Autodesk Inventor part; units mm, degrees
ref_plane "YZ Plane" through (0, 0, 0) normal (1, 0, 0) x (0, 1, 0)
ref_plane "XZ Plane" through (0, 0, 0) normal (0, 1, 0) x (-1, 0, 0)
ref_plane "XY Plane" through (0, 0, 0) normal (0, 0, 1) x (1, 0, 0)
sketch "Sketch1" plane through (0, 0, 0) normal (0, 1, 0) x (-1, 0, 0)
  circle A0 centre (0, 0) radius 12.7
  dimension "d0" = 25.4
extrude "Extrusion1" add sketch "Sketch1" along normal blind 3
sketch "Sketch2" plane through (0, 3, 0) normal (0, 1, 0) x (1, 0, 0)
  circle A0 centre (0, 0) radius 7.125
  dimension "d3" = 14.25
extrude "Extrusion2" add sketch "Sketch2" along normal blind 3
sketch "Sketch3" plane through (0, 6, 0) normal (0, 1, 0) x (1, 0, 0)
  circle A0 centre (0, 0) radius 2.54
  dimension "d6" = 5.08
extrude "Extrusion3" cut sketch "Sketch3" against normal up to next
properties part number "PhotonCerberCageInsert"
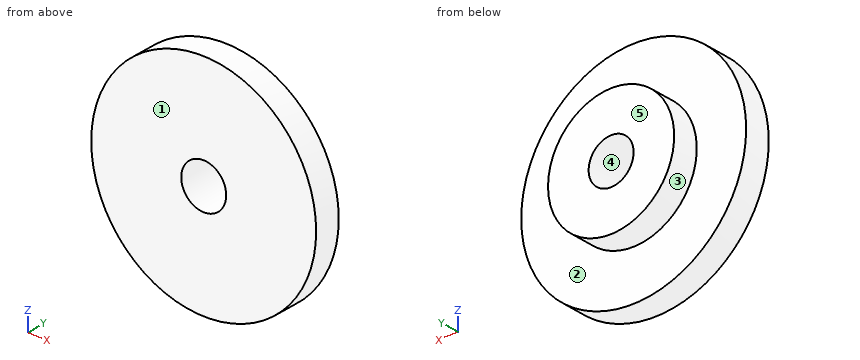
Geometry: final body of the model. Coordinates: model frame, mm. Face numbers are marked on the shaded views. A direction names the side the tool comes from. Give positions to 0.01 mm unless a question says otherwise; leave off trailing zeros. Write each loop counter-clockwise with the first axis right and the second up, starting at its lowest first coordinate (ties: lowest second). Pieces come first, ordered by that corner, then holes. Notation, with made-up numbers: (-22.75, -10.5) -> (21.25, -10.5) arc R6 cw to (21.25, -6.5) -> close; hole circle Ø6 at (-3, 14.25). An arc over 180 degrees is marked (long way). Answer as a JSON object with one key per item and string values.
1. Cut plane C-C on y = 2.5. Output: boundary loops of the cut face in (x, z).
Ans:
{"outline": "circle Ø25.4 at (0, 0); hole circle Ø5.08 at (0, 0)"}
2. Mould query, pull axis X, two halves, no side actions, for the marked faces 3, 4 and 5. Classes: pulls with the +X half, pulls with the -X half, needs draft (parallel to the pull), parting line crosses it, or undercut.
Ans:
{"face 3": "parting line crosses it", "face 4": "undercut", "face 5": "needs draft"}
3. Cut plane D-D on z = 5.5. Output: boundary loops of the cut face in (x, y), and give its area (3 significant figures).
Ans:
{"outline": "(-11.45, 0) -> (11.45, 0) -> (11.45, 3) -> (4.53, 3) -> (4.53, 6) -> (-4.53, 6) -> (-4.53, 3) -> (-11.45, 3) -> close", "area": "95.9 mm^2"}
4. Cut plane B-B on x = -1.5. Output: boundary loops of the cut face in (y, z).
Ans:
{"outline": "(0, -12.61) -> (3, -12.61) -> (3, -6.97) -> (6, -6.97) -> (6, -2.05) -> (0, -2.05) -> close; (0, 2.05) -> (6, 2.05) -> (6, 6.97) -> (3, 6.97) -> (3, 12.61) -> (0, 12.61) -> close"}
5. Contact query for a flat-ended pin moving along its axis: pin 1 (2 mm diameter, centred on x = -4, y = 2.5, fed in from +Z). Output: stop coordinate, or through.
Ans:
{"pin 1": "stops at z = 12.34"}
6. Ray query, probe 1 along Z at (x, y) = (0, 4.7) (3 decimals); probe 2 along Z at (x, y) = (0, 2.2). Return the intervals inside material, ascending. Write a range as from..to.
Ans:
{"probe 1": "z = -7.125..-2.54, 2.54..7.125", "probe 2": "z = -12.7..-2.54, 2.54..12.7"}
7. Cut plane A-A on z = 0. Output: boundary loops of the cut face in (x, y) (3 decimals), and give its area (3 significant figures).
Ans:
{"outline": "(-12.7, 0) -> (-2.54, 0) -> (-2.54, 6) -> (-7.125, 6) -> (-7.125, 3) -> (-12.7, 3) -> close; (2.54, 0) -> (12.7, 0) -> (12.7, 3) -> (7.125, 3) -> (7.125, 6) -> (2.54, 6) -> close", "area": "88.5 mm^2"}
8. Access query for the marked faces 1 and 2. Directions: +Z, -Z, +X, -X, +Y, -Y. A direction counts if a zero-diameter tool reaches every point of the face in a straight line with its end or side. Return the directions, or none.
Ans:
{"face 1": "+Z, -Z, +X, -X, -Y", "face 2": "+Y"}
